```python
from build123d import *

# Parameters (mm, degrees)
F1_DEPTH = 7
F2_START = 1.1
F2_DEPTH = 4.9


with BuildPart() as f1:
    # F0 (on Top) → F1 (new body)
    with BuildSketch(Plane.XY):
        Polygon((-7.4115242199, 14.465439185), (0, 11.15), (0, 40), align=None)
        Polygon((0, 40), (0, 11.15), (7.2415005954, 15.0512132379), align=None)
        Polygon((-40, 0), (-11.6101847588, 0), (-15.5867241284, 6.8052006492), align=None)
        Polygon((-15.2432164393, -7.1857707793), (-11.6101847588, 0), (-40, 0), align=None)
        Polygon((0, -40), (0, -11.6101847588), (-7.1857707793, -15.2432164393), align=None)
        Polygon((7.1857707793, -15.2432164393), (0, -11.6101847588), (0, -40), align=None)
        Polygon((40, 0), (11.6101847588, 0), (15.2432164393, -7.1857707793), align=None)
        Polygon((15.0074665088, 6.9666687107), (11.6101847588, 0), (40, 0), align=None)
        with BuildLine():
            ThreePointArc((-5.7679465413, 9.5421849016), (-2.9939220387, 10.7405274929), (0, 11.15))
            Line((0, 11.15), (-7.4115242199, 14.465439185))
            Line((-7.4115242199, 14.465439185), (-9.1110031263, 8.6103078786))
            Line((-9.1110031263, 8.6103078786), (-5.7679465413, 9.5421849016))
        make_face()
        Polygon((10.7080552853, 3.1080624202), (11.6101847588, 0), (15.0074665088, 6.9666687107), (9.1110031263, 8.6103078786), align=None)
        Polygon((-10.7080552332, -3.1080625996), (-11.6101847588, 0), (-15.2432164393, -7.1857707793), (-8.9983671347, -8.9983671347), align=None)
        Polygon((-7.1857707793, -15.2432164393), (0, -11.6101847588), (-3.1080626541, -10.7080552174), (-8.9983671347, -8.9983671347), align=None)
        Polygon((7.1857707793, -15.2432164393), (8.9983671347, -8.9983671347), (3.1080623688, -10.7080553002), (0, -11.6101847588), align=None)
        Polygon((15.2432164393, -7.1857707793), (11.6101847588, 0), (10.708055209, -3.1080626829), (8.9983671347, -8.9983671347), align=None)
        with BuildLine():
            Line((7.2415005954, 15.0512132379), (0, 11.15))
            ThreePointArc((0, 11.15), (2.9939220387, 10.7405274929), (5.7679465413, 9.5421849016))
            Line((5.7679465413, 9.5421849016), (8.8026408844, 8.6962638535))
            Line((8.8026408844, 8.6962638535), (9.02027697, 8.9228822539))
            Line((9.02027697, 8.9228822539), (7.2415005954, 15.0512132379))
        make_face()
        Polygon((-15.5867241284, 6.8052006492), (-11.6101847588, 0), (-10.7080552075, 3.108062688), (-9.1374538419, 8.5191785256), (-9.2095170056, 8.5828471347), align=None)
        with BuildLine():
            ThreePointArc((-10.7080552075, 3.108062688), (-9.6869346026, 5.5213945707), (-8.1307635844, 7.6297564532))
            Line((-8.1307635844, 7.6297564532), (-9.1374538419, 8.5191785256))
            Line((-9.1374538419, 8.5191785256), (-10.7080552075, 3.108062688))
        make_face()
        with BuildLine():
            ThreePointArc((5.7679465413, 9.5421849016), (6.9155239519, 8.7463151367), (7.9546122238, 7.813235205))
            Line((7.9546122238, 7.813235205), (8.8026408844, 8.6962638535))
            Line((8.8026408844, 8.6962638535), (5.7679465413, 9.5421849016))
        make_face()
        with BuildLine():
            ThreePointArc((-8.1307635844, 7.6297564532), (-7.0148329583, 8.6668690176), (-5.7679465413, 9.5421849016))
            Line((-5.7679465413, 9.5421849016), (-9.1110031263, 8.6103078786))
            Line((-9.1110031263, 8.6103078786), (-9.1374538419, 8.5191785256))
            Line((-9.1374538419, 8.5191785256), (-8.1307635844, 7.6297564532))
        make_face()
        with BuildLine():
            ThreePointArc((7.9546122238, 7.813235205), (9.6233285495, 5.631522674), (10.7080552853, 3.1080624202))
            Line((10.7080552853, 3.1080624202), (9.1110031263, 8.6103078786))
            Line((9.1110031263, 8.6103078786), (8.8026408844, 8.6962638535))
            Line((8.8026408844, 8.6962638535), (7.9546122238, 7.813235205))
        make_face()
        with BuildLine():
            Line((8.9983671347, -8.9983671347), (7.8842406102, -7.8842406102))
            ThreePointArc((7.8842406102, -7.8842406102), (5.6746069068, -9.5979860624), (3.1080623688, -10.7080553002))
            Line((3.1080623688, -10.7080553002), (8.9983671347, -8.9983671347))
        make_face()
        with BuildLine():
            Line((8.9983671347, -8.9983671347), (10.708055209, -3.1080626829))
            ThreePointArc((10.708055209, -3.1080626829), (9.5979859792, -5.6746070475), (7.8842406102, -7.8842406102))
            Line((7.8842406102, -7.8842406102), (8.9983671347, -8.9983671347))
        make_face()
        with BuildLine():
            Line((-8.9983671347, -8.9983671347), (-3.1080626541, -10.7080552174))
            ThreePointArc((-3.1080626541, -10.7080552174), (-5.6746070346, -9.5979859868), (-7.8842406102, -7.8842406102))
            Line((-7.8842406102, -7.8842406102), (-8.9983671347, -8.9983671347))
        make_face()
        with BuildLine():
            ThreePointArc((-7.8842406102, -7.8842406102), (-9.5979860012, -5.6746070102), (-10.7080552332, -3.1080625996))
            Line((-10.7080552332, -3.1080625996), (-8.9983671347, -8.9983671347))
            Line((-8.9983671347, -8.9983671347), (-7.8842406102, -7.8842406102))
        make_face()
        with BuildLine():
            ThreePointArc((-10.7080552332, -3.1080625996), (-11.0034097906, -1.8020746324), (-11.1400855815, -0.4700991772))
            Line((-11.1400855815, -0.4700991772), (-11.6101847588, 0))
            Line((-11.6101847588, 0), (-10.7080552332, -3.1080625996))
        make_face()
        with BuildLine():
            ThreePointArc((-11.1400855815, -0.4700991772), (-11.1475211198, -0.2351018567), (-11.15, 0))
            Line((-11.15, 0), (-11.6101847588, 0))
            Line((-11.6101847588, 0), (-11.1400855815, -0.4700991772))
        make_face()
        with BuildLine():
            Line((-11.6101847588, 0), (-11.15, 0))
            ThreePointArc((-11.15, 0), (-11.147721628, 0.22539411), (-11.1408874431, 0.4506961068))
            Line((-11.1408874431, 0.4506961068), (-11.6101847588, 0))
        make_face()
        with BuildLine():
            Line((-11.6101847588, 0), (-11.1408874431, 0.4506961068))
            ThreePointArc((-11.1408874431, 0.4506961068), (-11.0049749216, 1.7924918343), (-10.7080552075, 3.108062688))
            Line((-10.7080552075, 3.108062688), (-11.6101847588, 0))
        make_face()
        with BuildLine():
            Line((11.6101847588, 0), (11.1400855815, -0.4700991772))
            ThreePointArc((11.1400855815, -0.4700991772), (11.0034097836, -1.8020746752), (10.708055209, -3.1080626829))
            Line((10.708055209, -3.1080626829), (11.6101847588, 0))
        make_face()
        with BuildLine():
            Line((11.6101847588, 0), (11.15, 0))
            ThreePointArc((11.15, 0), (11.1475211198, -0.2351018567), (11.1400855815, -0.4700991772))
            Line((11.1400855815, -0.4700991772), (11.6101847588, 0))
        make_face()
        with BuildLine():
            ThreePointArc((11.1408874431, 0.4506961068), (11.147721628, 0.22539411), (11.15, 0))
            Line((11.15, 0), (11.6101847588, 0))
            Line((11.6101847588, 0), (11.1408874431, 0.4506961068))
        make_face()
        with BuildLine():
            ThreePointArc((10.7080552853, 3.1080624202), (11.004974944, 1.7924916967), (11.1408874431, 0.4506961068))
            Line((11.1408874431, 0.4506961068), (11.6101847588, 0))
            Line((11.6101847588, 0), (10.7080552853, 3.1080624202))
        make_face()
        Polygon((8.8026408844, 8.6962638535), (9.1110031263, 8.6103078786), (9.02027697, 8.9228822539), align=None)
        with BuildLine():
            Line((0, -11.6101847588), (-0.4700991772, -11.1400855815))
            ThreePointArc((-0.4700991772, -11.1400855815), (-1.8020746604, -11.003409786), (-3.1080626541, -10.7080552174))
            Line((-3.1080626541, -10.7080552174), (0, -11.6101847588))
        make_face()
        with BuildLine():
            ThreePointArc((0.4700991772, -11.1400855815), (0.2351018567, -11.1475211198), (0, -11.15))
            Line((0, -11.15), (0, -11.6101847588))
            Line((0, -11.6101847588), (0.4700991772, -11.1400855815))
        make_face()
        with BuildLine():
            ThreePointArc((3.1080623688, -10.7080553002), (1.8020745138, -11.00340981), (0.4700991772, -11.1400855815))
            Line((0.4700991772, -11.1400855815), (0, -11.6101847588))
            Line((0, -11.6101847588), (3.1080623688, -10.7080553002))
        make_face()
        with BuildLine():
            Line((0, -11.6101847588), (0, -11.15))
            ThreePointArc((0, -11.15), (-0.2351018567, -11.1475211198), (-0.4700991772, -11.1400855815))
            Line((-0.4700991772, -11.1400855815), (0, -11.6101847588))
        make_face()
    extrude(amount=F1_DEPTH)

    # F0 (on Top) → F2 (join)
    with BuildSketch(Plane.XY.offset(F2_START)):
        Polygon((-9.2095170056, 8.5828471347), (-24.540269553, 22.1277380295), (-15.5867241284, 6.8052006492), align=None)
        Polygon((-9.1110031263, 8.6103078786), (-7.4115242199, 14.465439185), (-24.540269553, 22.1277380295), (-9.2095170056, 8.5828471347), align=None)
        Polygon((23.1218005728, 23.6064064161), (7.2415005954, 15.0512132379), (9.02027697, 8.9228822539), align=None)
        Polygon((9.1110031263, 8.6103078786), (15.0074665088, 6.9666687107), (23.1218005728, 23.6064064161), (9.02027697, 8.9228822539), align=None)
        Polygon((23.482761909, -23.482761909), (15.2432164393, -7.1857707793), (8.9983671347, -8.9983671347), align=None)
        Polygon((23.482761909, -23.482761909), (8.9983671347, -8.9983671347), (7.1857707793, -15.2432164393), align=None)
        Polygon((-23.482761909, -23.482761909), (-7.1857707793, -15.2432164393), (-8.9983671347, -8.9983671347), align=None)
        Polygon((-8.9983671347, -8.9983671347), (-15.2432164393, -7.1857707793), (-23.482761909, -23.482761909), align=None)
    extrude(amount=F2_DEPTH)


solid = f1.part
```
Geometry check sheet. Reference: the model listing, model coordinates, mm. A direction names the side the tool comes from. Coordinates: 2 decimals unless noted, no trailing zeros. Write each loop counter-clockwise with the first axis right and the second up, starting at its lowest first coordinate (ties: lowest second). Pieces come first, ordered by that corner, then holes. Notation, with made-up numbers: M 52.5,60 L 70.5,60 A17 ccw 70.5,73 Z; hole C 86.5,-34.5 d7. An arc over 180 degrees is marked long. Answer as a JSON object with one key per item and string values.
1. Section check D-D, the plane x = 33.5. Enter the section's corners in (y, z), plus the area to 3 significant figures.
Answers below:
{"outline": "M -1.89,0 L 1.81,0 L 1.81,7 L -1.89,7 Z", "area": "25.9 mm²"}
2. Section check C-C, the plane y = 19. Enter the section's corners in (x, z).
Answers below:
{"outline": "M -22.71,1.1 L -17.55,1.1 L -17.55,6 L -22.71,6 Z; M -6.1,0 L 6.1,0 L 6.1,7 L -6.1,7 Z; M 14.57,1.1 L 20.88,1.1 L 20.88,6 L 14.57,6 Z"}
3. Tool access check on faces 1 (the flat face through (-15, -15, 1.1)), 2 (the flat face through (15, -15, 6)), 3 (the flat face through (15, 15, 1.1)), 4 (the flat face through (15.293, 19.389, 3.516)). Record the directions out of +Z, -Z, +X, -X, +Y, -Y that give a thin tool (end or side, any length) a straight path to the whole face; none if there is none.
Answers below:
{"face 1": "-Z, -X, -Y", "face 2": "+Z, +X, -Y", "face 3": "-Z, +X, +Y", "face 4": "+Z, -Z, +Y"}
4. Section check B-B, the plane z = 5. Enter the section's corners in (x, y), plus the area to 3 significant figures.
Answers below:
{"outline": "M -40,0 L -15.24,-7.19 L -23.48,-23.48 L -7.19,-15.24 L 0,-40 L 7.19,-15.24 L 23.48,-23.48 L 15.24,-7.19 L 40,0 L 15.01,6.97 L 23.12,23.61 L 7.24,15.05 L 0,40 L -7.41,14.47 L -24.54,22.13 L -15.59,6.81 Z; hole C 0,0 d22.3; hole M -9.21,8.58 L -9.14,8.52 L -9.11,8.61 Z", "area": "1,500 mm²"}
5. Go/stop test with flat-tipped pins: pin 1 Ø5 at (x, y) = (-19.5, -17.5) entering from +Z; pin 2 Ø12 at (x, y) = (-15, -15) entering from -Z; pin 3 Ø4 at (x, z) = (-15, 2) entering from -Y; pin 4 Ø6 at (x, y) = (-8.5, 22.5) entering from -Z. Record where each tip stops, or that it passes through.
Answers below:
{"pin 1": "stops at z = 6", "pin 2": "stops at z = 1.1", "pin 3": "stops at y = -20.21", "pin 4": "passes through"}
6. Scan lines: L1, parallel to Y at x = -18, z = 5.25; L2, parallel to X at y = -22, z = 5.25; L3, parallel to Y at x = 9.5, z = 4. Record each from-to range of solid material in increasing order.
Answers below:
{"L1": "y = -20.71 to -12.64, -6.39 to 6.13, 10.94 to 19.2", "L2": "x = -22.73 to -20.55, -5.22 to 5.22, 20.55 to 22.73", "L3": "y = -16.41 to -5.84, 5.84 to 16.27"}
7. Draft check along Y on faces 5 (the flat face through (15, 15, 6)), 6 (the flat face through (-15.856, 18.243, 3.516)), 7 (the flat face through (19.01, 15.17, 3.52)). Enter one of: released by +Y, released by -Y, zero draft, split by the parting line, or undercut.
Answers below:
{"face 5": "zero draft", "face 6": "released by +Y", "face 7": "undercut"}
8. Section check A-A, the plane y = -22. Enter the section's corners in (x, z), plus the area to 3 significant figures.
Answers below:
{"outline": "M -22.73,1.1 L -20.55,1.1 L -20.55,6 L -22.73,6 Z; M -5.22,0 L 5.22,0 L 5.22,7 L -5.22,7 Z; M 20.55,1.1 L 22.73,1.1 L 22.73,6 L 20.55,6 Z", "area": "94.5 mm²"}
